Job drawing, mm, ordinate dimensions from the low corner. One solid piece. Give positions to 0.01 mm unless a question says otherwise; leave off trailing zeros. Order: outer loops, then holes, each group sorted by start corner. A loop starts at its lowest first (then second) coordinate and runs counter-clockwise, first axis right, second up. Notation, with made-up numbers: (34.25, -36.5) -> (55.25, -36.5) arc R20 ccw to (55.25, -0.5) -> close; hole circle Ø4 at (57.25, 5). An arc over 180 degrees is marked (long way). Write item = value, one per line. Start each with the question number.
(1) Saw through at B-B, the plane y = 4. State how many separate pieces and enclosed holes the cut face has.
(2) Flat gauge pins, fed straight in: pin 1 (1 mm diameter, centred on x = 10, z = 25.5, fed in from -Y); pin 2 (2.5 mm diameter, centred on x = 91.61, z = 2.4, fed in from +Y); pin 3 (2 mm diameter, centred on y = 6.5, z = 10.5, fed in from +X). Where does each tip first touch, or does it go through?
(3) Saw through at A-A, the plane x = 82.5. List the corners of the cut face in (y, z).
(4) Saw through at D-D, the plane x = 52. List the corners of the cut face in (y, z).
(5) Probe line 1 along X through (y, z) = (3.5, 22.5) (1 decimal); line 2 along Z through (x, y) = (87, 7.5); line 3 along Y through (x, z) = (62, 24.25). List the from-to ranges inside material, lowest first. Write a range as from..to.
(6) Saw through at C-C, the plane z = 16.5. List the corners of the cut face in (x, y).
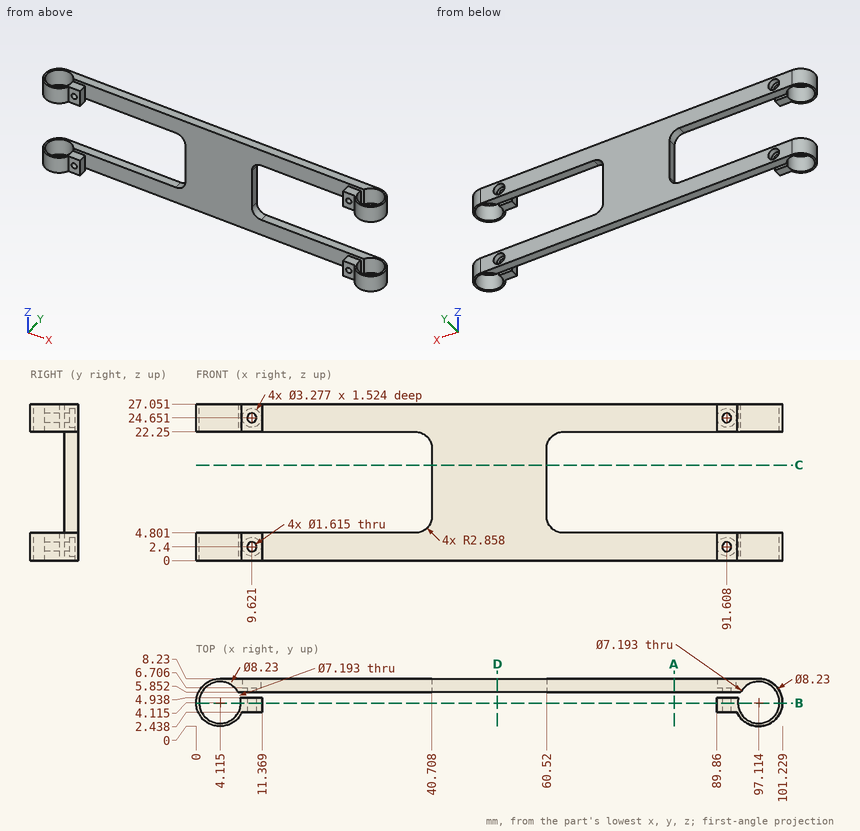
Results list:
q1.separate_pieces = 8
q1.enclosed_holes = 4
q2.pin_1 = 2.44
q2.pin_2 = 6.71
q2.pin_3 = 60.52
q3.outline = (5.85, 0) -> (8.23, 0) -> (8.23, 4.8) -> (5.85, 4.8) -> close; (5.85, 22.25) -> (8.23, 22.25) -> (8.23, 27.05) -> (5.85, 27.05) -> close
q4.outline = (5.85, 0) -> (8.23, 0) -> (8.23, 27.05) -> (5.85, 27.05) -> close
q5.line_1 = 0..0.6, 7.7..11.4, 89.9..93.6, 100.7..101.2
q5.line_2 = 0..4.8, 22.25..27.05
q5.line_3 = 5.85..8.23
q6.outline = (40.71, 5.85) -> (60.52, 5.85) -> (60.52, 8.23) -> (40.71, 8.23) -> close
